```python
from build123d import *

# Parameters (mm, degrees)
SKETCH1_W           = 13.97
SKETCH1_H           = 12.7
BOSS_EXTRUDE1_DEPTH = 2.54
FILLET1_R           = 0.635
SHELL1_START        = 0.635
SHELL1_OUTLINE_W    = 1.905
SHELL1_OUTLINE_H    = 11.43
SHELL1_DEPTH        = 12.7
SKETCH2_R           = 2.54
BOSS_EXTRUDE2_DEPTH = 1.905
BOSS_EXTRUDE3_DEPTH = 0.00254


# Read off the part's stored shape, not the designer's step: Shell1
with BuildPart() as part:
    # Sketch1 → Boss-Extrude1 (new body)
    with BuildSketch(Plane(origin=(0, 0, 0), x_dir=(1, 0, 0), z_dir=(0, 1, 0))):
        with Locations((6.985, 6.35)):
            Rectangle(SKETCH1_W, SKETCH1_H)
    extrude(amount=BOSS_EXTRUDE1_DEPTH)

    # Fillet1
    fillet1_edges = [part.edges().sort_by_distance(p)[0] for p in [
        (0, 1.27, -12.7),
        (13.97, 1.27, -12.7),
        (13.97, 1.27, 0),
        (0, 1.27, 0),
    ]]
    fillet(fillet1_edges, radius=FILLET1_R)

    # Shell1 outline → Shell1 (cut)
    with BuildSketch(Plane.YZ.offset(SHELL1_START)):
        with Locations((0.9525, -6.35)):
            Rectangle(SHELL1_OUTLINE_W, SHELL1_OUTLINE_H)
    extrude(amount=SHELL1_DEPTH, mode=Mode.SUBTRACT)

    # Sketch2 → Boss-Extrude2 (add)
    with BuildSketch(Plane(origin=(0, 1.905, 0), x_dir=(-1, 0, 0), z_dir=(0, -1, 0))):
        with Locations(Location((-6.985, 6.35, 0), (0, 0, 270))):
            Circle(SKETCH2_R)
    extrude(amount=BOSS_EXTRUDE2_DEPTH)

    # Sketch3 → Boss-Extrude3 (add)
    with BuildSketch(Plane(origin=(0, 2.54, 0), x_dir=(1, 0, 0), z_dir=(0, 1, 0))):
        Polygon((4.938346154, 8.001), (6.485141026, 8.001), (6.485141026, 7.431128205), (5.508217949, 7.431128205), (5.508217949, 6.820551282), (6.485141026, 6.820551282), (6.485141026, 6.250679487), (5.508217949, 6.250679487), (5.508217949, 4.826), (4.938346154, 4.826), align=None)
        with BuildLine():
            Line((6.973602564, 7.146192308), (7.543474359, 7.146192308))
            Line((7.543474359, 7.146192308), (7.543474359, 6.900689503))
            add(Edge.make_bspline(
                [(7.543474359, 6.900689503), (7.575985262, 6.925977153), (7.638119919, 6.974306769), (7.732575324, 7.035927275), (7.821729533, 7.086361185), (7.907569887, 7.124723797), (7.991711475, 7.152324047), (8.075517031, 7.172153181), (8.160234588, 7.18485032), (8.217185351, 7.18621543), (8.245637821, 7.186897436)],
                knots=[0, 0, 0, 0, 1.276643801, 2.439914479, 3.493451431, 4.44993799, 5.350072675, 6.235028322, 7.118224225, 8, 8, 8, 8], degree=3))
            add(Edge.make_bspline(
                [(8.245637821, 7.186897436), (8.274499022, 7.186118044), (8.331155985, 7.184588033), (8.41458024, 7.173886845), (8.494284014, 7.154396591), (8.57116351, 7.128518806), (8.644436227, 7.094361613), (8.714999799, 7.053805489), (8.781338547, 7.004405385), (8.822192885, 6.966784638), (8.842858373, 6.947754808)],
                knots=[0, 0, 0, 0, 1.048836932, 2.058954983, 3.049370783, 4.026390553, 5.001981509, 5.982488534, 6.97947532, 8, 8, 8, 8], degree=3))
            add(Edge.make_bspline(
                [(8.842858373, 6.947754808), (8.859432856, 6.93011972), (8.892703126, 6.894720476), (8.934569582, 6.834143303), (8.970495709, 6.768103097), (8.999932179, 6.695838062), (9.021684544, 6.616951149), (9.038418936, 6.532395199), (9.047808895, 6.441696762), (9.048968129, 6.379387791), (9.049564103, 6.347354167)],
                knots=[0, 0, 0, 0, 0.889584746, 1.785680191, 2.700364693, 3.65222533, 4.649950538, 5.707241244, 6.821271309, 8, 8, 8, 8], degree=3))
            Line((9.049564103, 6.347354167), (9.049564103, 4.826))
            Line((9.049564103, 4.826), (8.479692308, 4.826))
            Line((8.479692308, 4.826), (8.479692308, 5.833451923))
            add(Edge.make_bspline(
                [(8.479692308, 5.833451923), (8.479571792, 5.86631325), (8.479340847, 5.929285883), (8.477567699, 6.019409185), (8.474105481, 6.10080223), (8.470949759, 6.173613213), (8.464753823, 6.237583603), (8.459166228, 6.293118384), (8.450592604, 6.339713739), (8.439436929, 6.389834035), (8.419956373, 6.443496978), (8.38971376, 6.500039753), (8.351346764, 6.548074101), (8.306422447, 6.587936766), (8.254990424, 6.619471791), (8.197672176, 6.641658645), (8.134774997, 6.655486038), (8.090948982, 6.656963488), (8.068188902, 6.657730769)],
                knots=[0, 0, 0, 0, 1.49886392, 2.872294502, 4.110984203, 5.214877267, 6.195405875, 7.042225351, 7.75923308, 8.355011229, 9.382752534, 10.352059385, 11.267231453, 12.171456522, 13.078624015, 14.003401117, 14.963110155, 16, 16, 16, 16], degree=3))
            add(Edge.make_bspline(
                [(8.068188902, 6.657730769), (8.038588461, 6.656229723), (7.980684244, 6.653293385), (7.896937378, 6.631150715), (7.820017276, 6.593492551), (7.75055244, 6.541381225), (7.689204465, 6.477043335), (7.638676644, 6.400313021), (7.597233451, 6.313042165), (7.579412262, 6.249320264), (7.570187099, 6.216334535)],
                knots=[0, 0, 0, 0, 0.984188326, 1.925263693, 2.85911992, 3.81709677, 4.80007086, 5.801799564, 6.862098548, 8, 8, 8, 8], degree=3))
            add(Edge.make_bspline(
                [(7.570187099, 6.216334535), (7.56789428, 6.205975146), (7.562780832, 6.182871626), (7.558575667, 6.143840753), (7.552725978, 6.097534401), (7.550534244, 6.043114556), (7.546723058, 5.980838765), (7.5453135, 5.910624637), (7.543901419, 5.83260985), (7.543621428, 5.778119486), (7.543474359, 5.749497596)],
                knots=[0, 0, 0, 0, 0.543362196, 1.211806945, 2.009705693, 2.934833164, 4.000995085, 5.207458376, 6.533175157, 8, 8, 8, 8], degree=3))
            Line((7.543474359, 5.749497596), (7.543474359, 4.826))
            Line((7.543474359, 4.826), (6.973602564, 4.826))
            Line((6.973602564, 4.826), (6.973602564, 7.146192308))
        make_face()
    extrude(amount=BOSS_EXTRUDE3_DEPTH)


solid = part.part
```
Model file for the job. Use its own axes, mm. A direction names the side the tool comes from. Coordinates: 2 decimals unless noted, no trailing zeros. Loops run counter-clockwise (first coordinate to the right, second up) from the corner with the lowest first, then second, coordinate; pieces in that order, holes last. Notation, with made-up numbers: M -22,-20.5 L 7,-20.5 A28 cw 7,-2.5 Z; hole C 63.5,-12 d7. An arc over 180 degrees is marked long. Use CSV: the item, a comma, the result in double quotes. Start each with the question number.
1. Two-plate mould, pull along Z, no slides. Class faces 1 (the cylindrical face through (5.268, 0.966, -8.222)), 2 (the flat face through (7, 0, -6)), 3 (the flat face through (7, 1, 0)): pulls with the +Z half, pulls with the -Z half, needs draft (parallel to the pull), parting line crosses it, or undercut.
2. Tool access for faces 4 (the flat face through (7, 1, -0.635)), 5 (the flat face through (7, 1, -12.7)): list every direction of +Z, -Z, +X, -X, +Y, -Y with a clear straight run to the whole face (end or side of a thin tool).
3. Band-saw the part on B-B, the plane z = -2.75. List the corners of the cut face in (x, y) (3 decimals).
4. Probe probe 1 along X at (y, z) = (0.4, -2.5) (3 decimals); probe 2 along Z at (x, y) = (7, 1.25) (3 decimals); probe 3 along Z at (x, y) = (4.25, 0.45) (3 decimals). List the from-to ranges inside material, lowest first. Write a range as [from, to].
5. Band-saw the part on A-A, the plane y = 1.7. List the corners of the cut face in (x, z) (3 decimals).
6. Band-saw the part on C-C, the plane x = 10.5. List the corners of the cut face in (y, z) (3 decimals), then the cut area to 3 significant figures.
7. Flat gauge pin, fed straight in: pin 1 (4 mm diameter, centred on x = 5, z = -11, fed in from +Y). Where does the tip first touch, or does it go through?
Entries:
1,face 1,"undercut"
1,face 2,"needs draft"
1,face 3,"pulls with the +Z half"
2,face 4,"-Y"
2,face 5,"-Z, +X, -X, +Y, -Y"
3,outline,"M 0,0 L 0.635,0 L 0.635,1.905 L 13.335,1.905 L 13.335,0 L 13.97,0 L 13.97,2.54 L 0,2.54 Z"
4,probe 1,"x = [0, 0.635], [13.335, 13.97]"
4,probe 2,"z = [-12.7, -12.065], [-8.89, -3.81], [-0.635, 0]"
4,probe 3,"z = [-12.7, -12.065], [-0.635, 0]"
5,outline,"M 0,-12.065 A0.635 ccw 0.635,-12.7 L 13.335,-12.7 A0.635 ccw 13.97,-12.065 L 13.97,-0.635 A0.635 ccw 13.335,0 L 0.635,0 A0.635 ccw 0,-0.635 Z; C 6.985,-6.35 d5.08; hole M 0.635,-12.065 L 13.335,-12.065 L 13.335,-0.635 L 0.635,-0.635 Z"
6,outline,"M 0,-12.7 L 2.54,-12.7 L 2.54,0 L 0,0 L 0,-0.635 L 1.905,-0.635 L 1.905,-12.065 L 0,-12.065 Z"
6,area,"10.5 mm2"
7,pin 1,"stops at y = 2.54"
